from build123d import *

# Parameters (mm, degrees)
SKETCH1_R           = 12
SKETCH1_R_2         = 6
BOSS_EXTRUDE1_DEPTH = 30
CUT_EXTRUDE1_DEPTH  = 30
FILLET1_R           = 10


with BuildPart() as part:
    # Sketch1 → Boss-Extrude1 (new, symmetric)
    # profile 1 of 2: a face of its own
    with BuildSketch(Plane.XY):
        with BuildLine():
            Line((44.05305559, 11.898167926), (-54.25694441, 24.787849846))
            ThreePointArc((-54.25694441, 24.787849846), (-82.50694441, 0), (-54.25694441, -24.787849846))
            Line((-54.25694441, -24.787849846), (44.05305559, -11.898167926))
            ThreePointArc((44.05305559, -11.898167926), (30.49305559, 0), (44.05305559, 11.898167926))
        make_face()
        with BuildLine():
            ThreePointArc((-33.488504763, 6.936465737), (-32.476597793, 11.582960804), (-28.034816833, 13.281328853))
            Line((-28.034816833, 13.281328853), (23.35105559, 6.543992359))
            ThreePointArc((23.35105559, 6.543992359), (29.09305559, 0), (23.35105559, -6.543992359))
            Line((23.35105559, -6.543992359), (-28.034816833, -13.281328853))
            ThreePointArc((-28.034816833, -13.281328853), (-32.476597793, -11.582960804), (-33.488504763, -6.936465737))
            ThreePointArc((-33.488504763, -6.936465737), (-32.50694441, 0), (-33.488504763, 6.936465737))
        make_face(mode=Mode.SUBTRACT)
        with BuildLine():
            ThreePointArc((-41.744391243, 8.691485355), (-70.234866471, -12.727922061), (-48.815459055, 15.762553167))
            Line((-48.815459055, 15.762553167), (-45.48612913, 19.091883092))
            Line((-45.48612913, 19.091883092), (-38.415061318, 12.02081528))
            Line((-38.415061318, 12.02081528), (-41.744391243, 8.691485355))
        make_face(mode=Mode.SUBTRACT)
    # profile 2 of 2: a face of its own
    with BuildSketch(Plane.XY):
        with Locations((42.49305559, 0)):
            Circle(SKETCH1_R)
        with Locations((42.49305559, 0)):
            Circle(SKETCH1_R_2, mode=Mode.SUBTRACT)
    extrude(amount=BOSS_EXTRUDE1_DEPTH, both=True)

    # Sketch5 → Cut-Extrude1 (cut, symmetric)
    with BuildSketch(Plane(origin=(0, 0, 0), x_dir=(1, 0, 0), z_dir=(0, 1, 0))):
        with BuildLine():
            ThreePointArc((-14.84129936, 10.479353549), (-21.329766336, 6.143898522), (-28.983434984, 4.621489173))
            Line((-28.983434984, 4.621489173), (-82.50694441, 4.621489173))
            Line((-82.50694441, 4.621489173), (-82.50694441, 30))
            Line((-82.50694441, 30), (4.679347091, 30))
            Line((4.679347091, 30), (-14.84129936, 10.479353549))
        make_face()
        with BuildLine():
            ThreePointArc((-28.983434984, -4.621489173), (-21.329766336, -6.143898522), (-14.84129936, -10.479353549))
            Line((-14.84129936, -10.479353549), (4.679347091, -30))
            Line((4.679347091, -30), (-82.50694441, -30))
            Line((-82.50694441, -30), (-82.50694441, -4.621489173))
            Line((-82.50694441, -4.621489173), (-28.983434984, -4.621489173))
        make_face()
    extrude(amount=CUT_EXTRUDE1_DEPTH, both=True, mode=Mode.SUBTRACT)

    # Fillet1
    fillet1_edges = [part.edges().sort_by_distance(p)[0] for p in [
        (4.679347091, 13.026323567, -30),
        (4.679347091, -13.026323567, -30),
        (4.679347091, -13.026323567, 30),
        (4.679347091, 13.026323567, 30),
    ]]
    fillet(fillet1_edges, radius=FILLET1_R)


solid = part.part
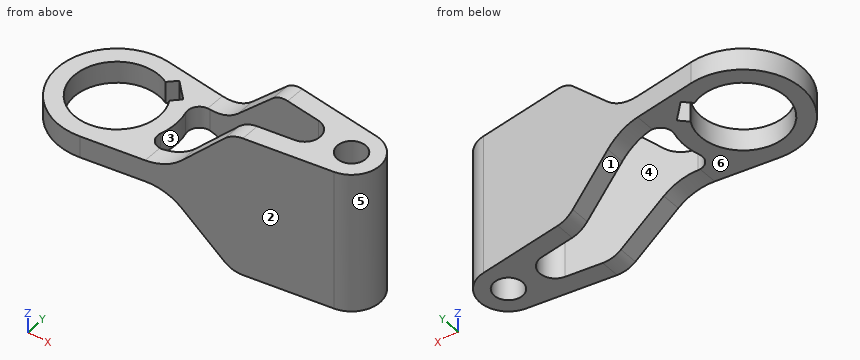
CAD build for the part. Positions are in the model's coordinates, mm. Face numbers are marked on the shaded views. A direction names the side the tool comes from. Round coordinates to 2 decimals unless told otherwise and drop trailing zeros. Order: outer loops, then holes, each group sorted by start corner. A loop starts at its lowest first (then second) coordinate and runs counter-clockwise, first axis right, second up. Notation, with made-up numbers: (18, 69.5) -> (62, 69.5) arc R9 cw to (62, 74.5) -> close; hole circle Ø10 at (-31, 1.5). An arc over 180 degrees is marked (long way). Write each question's results on one line, items separated by ' | '.
1. Cut at A-A (y = 0). Give the cut face in (x, z).
Findings below:
outline: (-82.51, -4.62) -> (-75.51, -4.62) -> (-75.51, 4.62) -> (-82.51, 4.62) -> close; (-39.51, -4.62) -> (-32.51, -4.62) -> (-32.51, 4.62) -> (-39.51, 4.62) -> close; (29.09, -30) -> (36.49, -30) -> (36.49, 30) -> (29.09, 30) -> close; (48.49, -30) -> (54.49, -30) -> (54.49, 30) -> (48.49, 30) -> close
2. Flat gauge pins, fed straight in: P1, Ø1, axis at x = 5.5, y = -14.5, coming from the +Z side; P2, Ø1.5, axis at x = 24.5, z = 8.5, coming from the +Y side; P3, Ø1.5, axis at x = 4.5, z = 21.5, coming from the -Y side. Where does each tip first touch, or does it go through?
Findings below:
P1: stops at z = 29.59 | P2: stops at y = 14.56 | P3: stops at y = -17.18
3. Cut at C-C (z = -22). Give the cut face in (x, y).
Findings below:
outline: (-3.32, -18.11) -> (44.05, -11.9) arc R12 ccw to (44.05, 11.9) -> (-3.32, 18.11) -> (-3.32, 10.04) -> (23.35, 6.54) arc R6.6 cw to (23.35, -6.54) -> (-3.32, -10.04) -> close; hole circle Ø12 at (42.49, 0)
4. Pull direction Y, two halves, no side cores. Call the marked faces 1, 2 and 3: pulls with the +Y half, pulls with the -Y half, needs draft (parallel to the pull), parting line crosses it, or undercut.
Findings below:
face 1: needs draft | face 2: pulls with the -Y half | face 3: undercut
5. Cut at B-B (x = -24.5). Give the cut face in (y, z).
Findings below:
outline: (-20.89, -5.13) -> (-12.82, -5.13) -> (-12.82, 5.13) -> (-20.89, 5.13) -> close; (12.82, -5.13) -> (20.89, -5.13) -> (20.89, 5.13) -> (12.82, 5.13) -> close
6. 3-axis set-ups, long thin cutter, end or side, ignore diameter. For the marked faces 4, 5 and 6: which of +Z, -Z, +X, -X, +Y, -Y reach the whole face in a straight line?
Findings below:
face 4: +Z, -Z | face 5: +Z, -Z, +X | face 6: -Z, -X, +Y, -Y
7. Wall check: line 1 along X through (y, z) = (-0.5, -11.5); line 2 along Z through (x, y) = (-56, 19.5); line 3 along X through (y, z) = (5, 10.5). Give the ranges that are in metal, low to high. Write a range as [from, to].
Findings below:
line 1: x = [29.07, 36.51], [48.47, 54.48] | line 2: z = [-4.62, 4.62] | line 3: x = [26.8, 39.18], [45.81, 53.4]
8. Cut at D-D (x = -59.5). Give the cut face in (y, z).
Findings below:
outline: (-24.92, -4.62) -> (-17.89, -4.62) -> (-17.89, 4.62) -> (-24.92, 4.62) -> close; (17.89, -4.62) -> (24.92, -4.62) -> (24.92, 4.62) -> (17.89, 4.62) -> close
